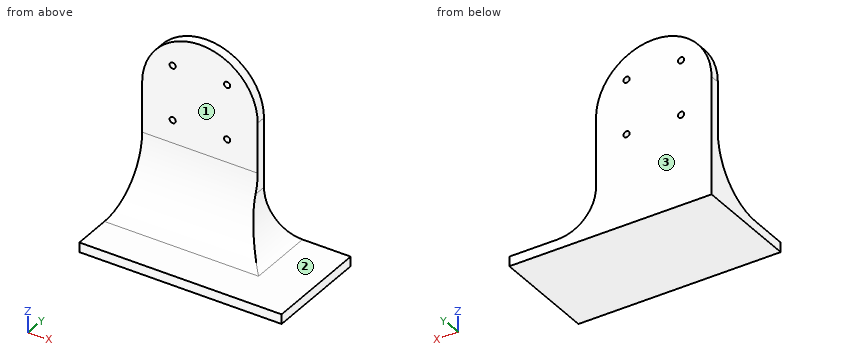
```python
from build123d import *

# Parameters (mm, degrees)
SKETCH1_R           = 30
SKETCH1_R_2         = 1.6
BOSS_EXTRUDE1_DEPTH = 5
BOSS_EXTRUDE2_DEPTH = 5
SKETCH3_W           = 60
SKETCH3_H           = 5
BOSS_EXTRUDE3_DEPTH = 50
FILLET1_R           = 30
SKETCH4_W           = 5
SKETCH4_H           = 55
BOSS_EXTRUDE4_DEPTH = 45
FILLET2_R           = 20


with BuildPart() as part:
    # Sketch1 → Boss-Extrude1 (new body)
    with BuildSketch(Plane(origin=(0, 0, 0), x_dir=(1, 0, 0), z_dir=(0, 1, 0))):
        with Locations(Location((0, 0, 0), (0, 0, 270))):
            Circle(SKETCH1_R)
        with Locations(Location((14.142135624, 14.142135624, 0), (0, 0, 270))):
            Circle(SKETCH1_R_2, mode=Mode.SUBTRACT)
        with Locations(Location((-14.142135624, 14.142135624, 0), (0, 0, 270))):
            Circle(SKETCH1_R_2, mode=Mode.SUBTRACT)
        with Locations(Location((-14.142135624, -14.142135624, 0), (0, 0, 270))):
            Circle(SKETCH1_R_2, mode=Mode.SUBTRACT)
        with Locations(Location((14.142135624, -14.142135624, 0), (0, 0, 270))):
            Circle(SKETCH1_R_2, mode=Mode.SUBTRACT)
    extrude(amount=BOSS_EXTRUDE1_DEPTH)

    # Sketch2 → Boss-Extrude2 (add)
    with BuildSketch(Plane.XZ):
        with BuildLine():
            Line((-30, -61), (30, -61))
            Line((30, -61), (30, 0))
            ThreePointArc((30, 0), (0, -30), (-30, 0))
            Line((-30, 0), (-30, -61))
        make_face()
    extrude(amount=-BOSS_EXTRUDE2_DEPTH)

    # Sketch3 → Boss-Extrude3 (add)
    with BuildSketch(Plane.XZ):
        with Locations((0, -58.5)):
            Rectangle(SKETCH3_W, SKETCH3_H)
    extrude(amount=BOSS_EXTRUDE3_DEPTH)

    # Fillet1
    fillet1_edges = [part.edges().sort_by_distance(p)[0] for p in [
        (0, 0, -56),
    ]]
    fillet(fillet1_edges, radius=FILLET1_R)

    # Sketch4 → Boss-Extrude4 (add)
    with BuildSketch(Plane(origin=(30, 0, 0), x_dir=(0, 0, -1), z_dir=(1, 0, 0))):
        with Locations((58.5, -22.5)):
            Rectangle(SKETCH4_W, SKETCH4_H)
    extrude(amount=BOSS_EXTRUDE4_DEPTH)

    # Fillet2
    fillet2_edges = [part.edges().sort_by_distance(p)[0] for p in [
        (30, -12.5, -56),
    ]]
    fillet(fillet2_edges, radius=FILLET2_R)


solid = part.part
```
Work out the finished part from the listing and answer in its coordinate system (mm). Face numbers are marked on the shaded views. A direction names the side the tool comes from. Give positions to 0.01 mm unless a question says otherwise; leave off trailing zeros. Loops run counter-clockwise (first coordinate to the right, second up) from the corner with the lowest first, then second, coordinate; pieces in that order, holes last. Notation, with made-up numbers: M -17.5,-0.75 L 36.5,-0.75 A29 ccw 36.5,26.25 Z; hole C 15,46 d3. An arc over 180 degrees is marked long. One line per item, written item: value. Start each with the question number.
1. Each of these flat-tipped pins is pushed along its axis until it touches: P1, Ø2.5, axis at x = 14.14, z = -14.14, coming from the -Y side; P2, Ø5, axis at x = 14.14, z = 14.14, coming from the +Y side; P3, Ø5.5, axis at y = 3, z = -19, coming from the +X side; P4, Ø1.5, axis at x = -10, z = -41, coming from the -Y side. Where does it stop, or does it pass through?
2. Find the intervals of material crossed by probe 1 along Z at (x, y) = (-8.5, -39); probe 2 along Y at (x, z) = (5.5, 6); probe 3 along Z at (x, y) = (0, 1), in increasing order.
3. Find section C-C (y = -21.5). Give the vertices of the cut face in (x, z).
4. Find section A-A (x = 0). Give the vertices of the cut face in (y, z), and give its area (3 significant figures).
5. Find section B-B (z = -6). Give the vertices of the cut face in (x, y).
6. Find section D-D (x = 19.5). Give the vertices of the cut face in (y, z), and give its area (3 significant figures).
7. Which of the six approach directions +Z, -Z, +X, -X, +Y, -Y give full straight-line access (tool end or side, diameter ignored) to the marked faces 1, 2 and 3?
Reported:
1. P1: passes through
1. P2: stops at y = 5
1. P3: stops at x = 30
1. P4: stops at y = -4.47
2. probe 1: z = -61 to -56
2. probe 2: y = 0 to 5
2. probe 3: z = -61 to 30
3. outline: M -30,-61 L 75,-61 L 75,-56 L 50,-56 A20 cw 43.1,-54.77 L -30,-54.77 Z
4. outline: M -50,-61 L 5,-61 L 5,30 L 0,30 L 0,-26 A30 cw -30,-56 L -50,-56 Z
4. area: 898 mm²
5. outline: M -30,0 L 30,0 L 30,5 L -30,5 Z
6. outline: M -50,-61 L 5,-61 L 5,22.8 L 0,22.8 L 0,-26 A30 cw -30,-56 L -50,-56 Z
6. area: 862 mm²
7. face 1: +Z, +X, -X, -Y
7. face 2: +Z, +X, -Y
7. face 3: +Z, -Z, +X, -X, +Y
